Geometry check sheet. Reference: the model listing, model coordinates, mm. Face numbers are marked on the shaded views. Round coordinates to 2 decimals unless told otherwise and drop trailing zeros. Loops run counter-clockwise (first coordinate to the right, second up) from the corner with the lowest first, then second, coordinate; pieces in that order, holes last. Notation, with made-up numbers: M 56,16 L 93,16 A16 ccw 93,42 Z; hole C 41,34 d7. An arc over 180 degrees is marked long. Write item = value, one per line.
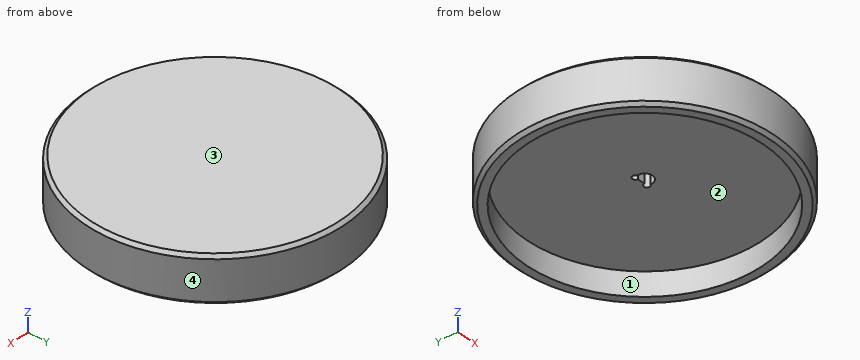
from build123d import *

# Parameters (mm, degrees)
F2_SIZE  = 1.27
F4_DEPTH = 7
F5_SIZE  = 1.27


with BuildPart() as f1:
    # F0 (on Front) → F1 (revolve)
    with BuildSketch(Plane.XZ):
        Polygon((0, 0), (0, 3.1056862596), (-50.8, 3.1056862596), (-50.8, -15), (-46.4363807935, -15), (-46.4363807935, -5.7271113946), (-1, -5.7271113946), (-1, 0), align=None)
    revolve(axis=Axis((0, 0, 4.3935226277), (0, 0, -1)))

    # F2
    f2_edges = [f1.edges().sort_by_distance(p)[0] for p in [
        (50.8, 0, 3.105686),
    ]]
    chamfer(f2_edges, length=F2_SIZE)

    # F3 (on face) → F4 (cut)
    with BuildSketch(Plane(origin=(0, 0, -5.7271113946), x_dir=(1, 0, 0), z_dir=(0, 0, -1))):
        with BuildLine():
            ThreePointArc((-2.9705407732, -0.4193894549), (-3.2616732298, -2.4306384889), (-1.4550762114, -1.5))
            Line((-1.4550762114, -1.5), (1.4550762114, -1.5))
            ThreePointArc((1.4550762114, -1.5), (3.2616732298, -2.4306384889), (2.9705407732, -0.4193894549))
            ThreePointArc((2.9705407732, -0.4193894549), (0, 3), (-2.9705407732, -0.4193894549))
        make_face()
    extrude(amount=-F4_DEPTH, mode=Mode.SUBTRACT)

    # F5
    f5_edges = [f1.edges().sort_by_distance(p)[0] for p in [
        (50.8, 0, -15),
    ]]
    chamfer(f5_edges, length=F5_SIZE)


solid = f1.part
(1) Sectioned sample at A-A on z = -8.25. Record the cut outline in (x, y).
Result set:
outline = C 0,0 d101.6; hole C 0,0 d92.87
(2) Sectioned sample at B-B on x = 0. Record the cut outline in (y, z).
Result set:
outline = M -50.8,-13.73 L -49.53,-15 L -46.44,-15 L -46.44,-5.73 L -3,-5.73 L -3,1.27 L 1.5,1.27 L 1.5,-5.73 L 46.44,-5.73 L 46.44,-15 L 49.53,-15 L 50.8,-13.73 L 50.8,1.84 L 49.53,3.11 L -49.53,3.11 L -50.8,1.84 Z
(3) Sectioned sample at C-C on z = -2.25. Record the cut outline in (x, y), then the cut area to 3 significant figures.
Result set:
outline = C 0,0 d101.6; hole M -2.97,0.42 A3 ccw long 2.97,0.42 A1.14 ccw long 1.46,1.5 L -1.46,1.5 A1.14 ccw long Z
area = 8,080 mm2
(4) Depth check by flat-ended pin: pin 1 Ø5 at (y, z) = (-25, -3) entering from -X; pin 2 Ø2 at (x, z) = (36.5, -7.5) entering from -Y; pin 3 Ø3 at (x, y) = (-0.5, -1.5) entering from -Z. Enter the tip coordinate at first touch or a pass-through.
Result set:
pin_1 = -45.55
pin_2 = -36.34
pin_3 = -5.73
(5) Release check for a two-part mould opening along Y. For the marked faces 1, 2, 3 and 4 record: released by +Y, released by -Y, zero draft, split by the parting line, or undercut.
Result set:
face_1 = undercut
face_2 = undercut
face_3 = zero draft
face_4 = split by the parting line
(6) Material ranges on line 1 along Y through (x, z) = (0, 0.25); line 2 along Z through (x, y) = (-23, 37.5); line 3 along X through (y, z) = (20, -8.75), recorded low to high. Write a range as from..to.
Result set:
line_1 = -50.8..-3, 1.5..50.8
line_2 = -5.73..3.11
line_3 = -46.7..-41.91, 41.91..46.7
